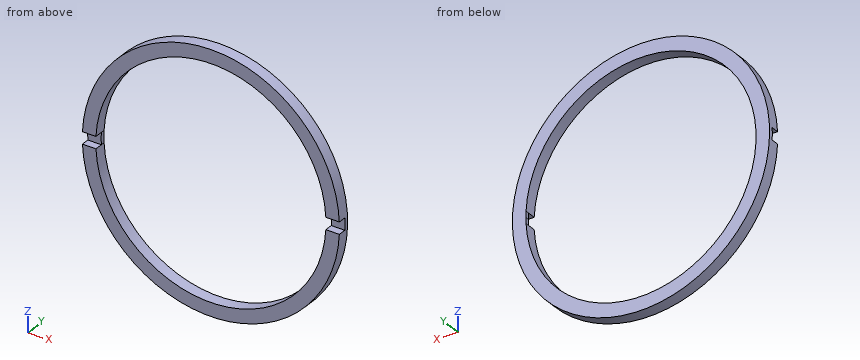
```python
from build123d import *

# Parameters (mm, degrees)
SKETCH_2_R          = 3.24
EXTRUDE_2_DEPTH     = 0.3
CUT_EXTRUDE_1_DEPTH = 0.6
SKETCH_4_W          = 7.550166352
SKETCH_4_H          = 0.3
CUT_EXTRUDE_2_DEPTH = 0.2


with BuildPart() as part:
    # Эскиз2 → Бобышка-Вытянуть2 (new body)
    with BuildSketch(Plane(origin=(0, 0, 0), x_dir=(1, 0, 0), z_dir=(0, 1, 0))):
        with Locations(Location((0, 0, 0), (0, 0, 270))):
            Circle(SKETCH_2_R)
    extrude(amount=EXTRUDE_2_DEPTH)

    # Эскиз3 → Вырез-Вытянуть1 (cut)
    with BuildSketch(Plane.XZ):
        with BuildLine():
            Line((-2.896118092, 0.15), (2.896118092, 0.15))
            ThreePointArc((2.896118092, 0.15), (0, 2.9), (-2.896118092, 0.15))
        make_face()
        with BuildLine():
            Line((-2.896118092, -0.15), (2.896118092, -0.15))
            ThreePointArc((2.896118092, -0.15), (2.89902936, -0.075025111), (2.9, 0))
            ThreePointArc((2.9, 0), (2.89902936, 0.075025111), (2.896118092, 0.15))
            Line((2.896118092, 0.15), (-2.896118092, 0.15))
            ThreePointArc((-2.896118092, 0.15), (-2.9, 0), (-2.896118092, -0.15))
        make_face()
        with BuildLine():
            ThreePointArc((-2.896118092, -0.15), (0, -2.9), (2.896118092, -0.15))
            Line((2.896118092, -0.15), (-2.896118092, -0.15))
        make_face()
    extrude(amount=-CUT_EXTRUDE_1_DEPTH, mode=Mode.SUBTRACT)

    # Эскиз4 → Вырез-Вытянуть2 (cut)
    with BuildSketch(Plane.XZ):
        Rectangle(SKETCH_4_W, SKETCH_4_H)
    extrude(amount=-CUT_EXTRUDE_2_DEPTH, mode=Mode.SUBTRACT)


solid = part.part
```
CAD build for the part. Positions are in the model's coordinates, mm. Round coordinates to 2 decimals unless told otherwise and drop trailing zeros. Write each loop counter-clockwise with the first axis right and the second up, starting at its lowest first coordinate (ties: lowest second). Pieces come first, ordered by that corner, then holes. Notation, with made-up numbers: (41, 40) - (63, 40) arc R22 cw to (63, 66) - close; hole circle Ø8 at (55, 56). An arc over 180 degrees is marked (long way). Write item = value, one per line. Start each with the question number.
Q1. Probe L1, parallel to X at y = 0.15, z = 0.5; L2, parallel to X at y = 0.25, z = 2.5; L3, parallel to Z at x = 2, y = 0.25. List the from-to ranges inside material, lowest first. Write a range as from..to.
Q2. Band-saw the part on B-B (y = 0.1). Give the cut face in (x, z), then the cut area to 3 significant figures.
Q3. Band-saw the part on A-A (x = 0). Give the cut face in (y, z).
Answers below:
q1.L1 = -3.2..-2.86, 2.86..3.2
q1.L2 = -2.06..-1.47, 1.47..2.06
q1.L3 = -2.55..-2.1, 2.1..2.55
q2.outline = (-3.24, -0.15) arc R3.24 ccw to (3.24, -0.15) - (2.9, -0.15) arc R2.9 cw to (-2.9, -0.15) - close; (-3.24, 0.15) - (-2.9, 0.15) arc R2.9 cw to (2.9, 0.15) - (3.24, 0.15) arc R3.24 ccw to start
q2.area = 6.35 mm2
q3.outline = (0, -3.24) - (0.3, -3.24) - (0.3, -2.9) - (0, -2.9) - close; (0, 2.9) - (0.3, 2.9) - (0.3, 3.24) - (0, 3.24) - close
